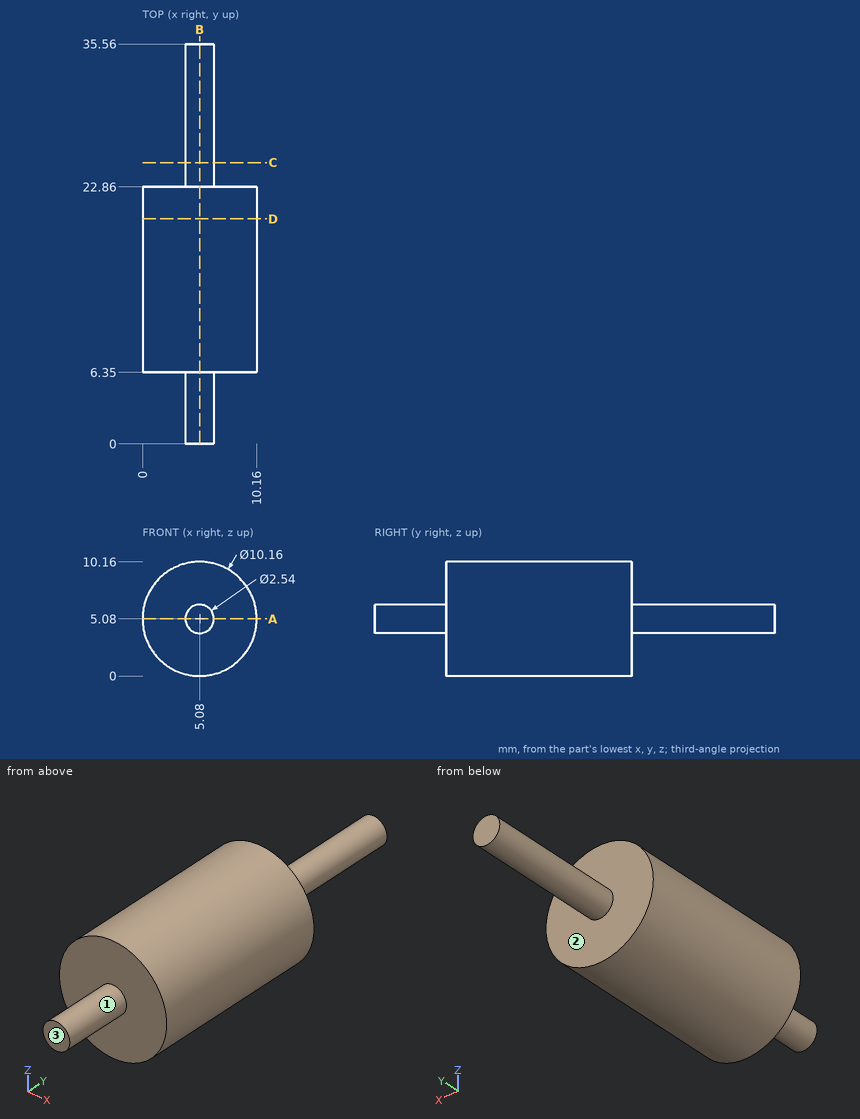
Source: three-view drawing plus pictorial views. Frame: mm from the lowest corner of the part. A direction names the side the tool comes from. Round coordinates to 2 decimals unless told otherwise and drop trailing zeros. Loops run counter-clockwise (first coordinate to the right, second up) from the corner with the lowest first, then second, coordinate; pieces in that order, holes last. Notation, with made-up numbers: M 51,-4.75 L 98,-4.75 A23 ccw 98,22.25 Z; hole C -35,22.5 d3. An arc over 180 degrees is marked long. Put each result on its own line as item: value.
(1) Section C-C, the plane y = 25. Return loops of the section in (x, z).
Solutions:
outline: C 5.08,5.08 d2.54
(2) Section A-A, the plane z = 5.08. Return loops of the section in (x, y), and give its area (3 significant figures).
Solutions:
outline: M 0,6.35 L 3.81,6.35 L 3.81,0 L 6.35,0 L 6.35,6.35 L 10.16,6.35 L 10.16,22.86 L 6.35,22.86 L 6.35,35.56 L 3.81,35.56 L 3.81,22.86 L 0,22.86 Z
area: 216 mm²
(3) Section B-B, the plane x = 5.08. Return loops of the section in (y, z).
Solutions:
outline: M 0,3.81 L 6.35,3.81 L 6.35,0 L 22.86,0 L 22.86,3.81 L 35.56,3.81 L 35.56,6.35 L 22.86,6.35 L 22.86,10.16 L 6.35,10.16 L 6.35,6.35 L 0,6.35 Z
(4) Section D-D, the plane y = 20. Return loops of the section in (x, z), and give its area (3 significant figures).
Solutions:
outline: C 5.08,5.08 d10.16
area: 81.1 mm²
(5) Ray query, line 1 (Y direction, x = 8.75, z = 5.75); line 2 (Z direction, x = 1.5, y = 21); line 3 (Z direction, x = 1.25, y = 10.5). Return the intervals inside material, ascending. Write a range as [from, to].
Solutions:
line 1: [6.35, 22.86]
line 2: [1.48, 8.68]
line 3: [1.74, 8.42]
(6) First-contact query: pin 1 (4 mm diameter, centred on y = 23.5, z = 5.5, fed in from -X); pin 2 (6 mm diameter, centred on y = 27, z = 5, fed in from -X); pin 3 (2 mm diameter, centred on y = 4.5, z = 5.5, fed in from +X). Flat tips, straight axial feed; report the tip coordinate or a pass-through.
Solutions:
pin 1: x = 0
pin 2: x = 3.81
pin 3: x = 6.35
(7) Access query for the marked faces 1, 2 and 3. Directions: +Z, -Z, +X, -X, +Y, -Y. A direction counts if a zero-diameter tool reaches every point of the face in a straight line with its end or side. Return the directions, or none.
Solutions:
face 1: -Y
face 2: +Y
face 3: +Z, -Z, +X, -X, -Y
